```python
from build123d import *

# Parameters (mm, degrees)
F0_R     = 3.175
F0_R_2   = 1.905
F1_DEPTH = 7.62


with BuildPart() as f1:
    # F0 (on Front) → F1 (new body)
    with BuildSketch(Plane.XZ):
        with BuildLine():
            Line((0, 50.8), (-24.807708, 5.453221))
            ThreePointArc((-24.807708, 5.453221), (15.916158, -19.794846), (0, 25.4))
            Line((0, 25.4), (0, 50.8))
        make_face()
        Circle(F0_R, mode=Mode.SUBTRACT)
        with Locations((-3.458634, 37.484073)):
            Circle(F0_R_2, mode=Mode.SUBTRACT)
    extrude(amount=F1_DEPTH)


solid = f1.part
```
CAD build for the part. Positions are in the model's coordinates, mm. Round coordinates to 2 decimals unless told otherwise and drop trailing zeros. Loops run counter-clockwise (first coordinate to the right, second up) from the corner with the lowest first, then second, coordinate; pieces in that order, holes last. Notation, with made-up numbers: M 13.5,84.5 L 20.5,84.5 A16 ccw 20.5,93.5 Z; hole C 1,-12 d4. An arc over 180 degrees is marked long. Return JSON: item names as keys, results as strings. Group by question number.
(1) Saw through at A-A, the plane z = 0. List the corners of the cut face in (x, y) (3 decimals).
(2) Drop flat-ended pins along their axis: P1, Ø1.5, axis at y = -5.5, z = 8, coming from the +X side; P2, Ø2, axis at y = -2, z = 6, coming from the -X side; P3, Ø2, axis at y = -1, z = 34, coming from the +X side. Give the stop position or say it passes through.
(3) Mould opens along Z. For faces 1 (the flat face through (-12.23, -3.757, 28.444)), 2 (the flat face through (0, -4, 38)), 3 (the cylindrical face through (-0.69, -3.76, -3.1)) say: +Z half, -Z half, draft (parallel to the pull), parting line (faces both ways), or undercut.
(4) Saw through at B-B, the plane y = -4.5. List the corners of the cut face in (x, z) (3 decimals), and give its area (3 significant figures).
(5) Saw through at C-C, the plane x = 5.5. List the corners of the cut face in (y, z).
(6) Wall check: probe 1 along Z at (x, y) = (-4.5, -4); probe 2 along X at (y, z) = (-2, 41.5); probe 3 along X at (y, z) = (-0.25, 6.5). Give the ranges that are in metal, low to high. Write a range as [from, to].
(7) Saw through at D-D, the plane z = 34. List the corners of the cut face in (x, y).
Answer list:
{
 "1": {"outline": "M -25.4,-7.62 L -3.175,-7.62 L -3.175,0 L -25.4,0 Z; M 3.175,-7.62 L 25.4,-7.62 L 25.4,0 L 3.175,0 Z"},
 "2": {"P1": "x = 24.34", "P2": "x = -24.9", "P3": "x = 0"},
 "3": {"face 1": "+Z half", "face 2": "draft", "face 3": "undercut"},
 "4": {"outline": "M -24.808,5.453 A25.4 ccw long 0,25.4 L 0,50.8 Z; hole C -3.459,37.484 d3.81; hole C 0,0 d6.35", "area": "2,180 mm2"},
 "5": {"outline": "M -7.62,-24.8 L 0,-24.8 L 0,24.8 L -7.62,24.8 Z"},
 "6": {"probe 1": "[-25, 35.89], [39.08, 42.57]", "probe 2": "[-5.09, 0]", "probe 3": "[-24.24, 24.55]"},
 "7": {"outline": "M -9.19,-7.62 L 0,-7.62 L 0,0 L -9.19,0 Z"}
}
